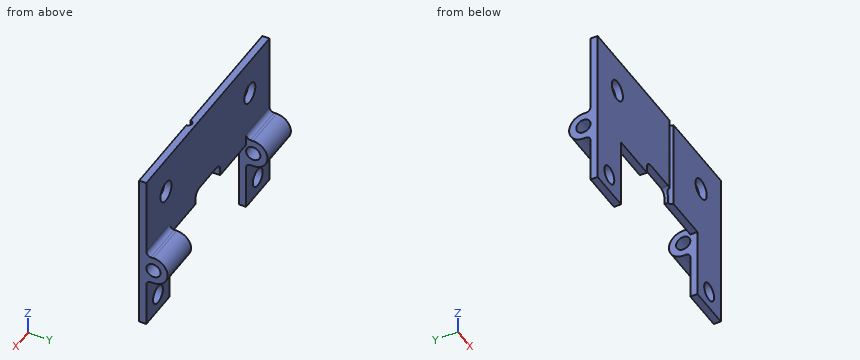
from build123d import *

# Parameters (mm, degrees)
SKETCH1_W                     = 25
SKETCH1_H                     = 10
BASE_PLATE_DEPTH              = 0.79
PINHOLDER_DEPTH               = 4.75
SKETCH4_R                     = 0.79
PIN_SHAFT_DEPTH               = 30.913269547
SKETCH5_R                     = 1.125
SCREW_HOLES_DEPTH             = 4
SKETCH11_R                    = 1
SET_SCREW_HOLE_DEPTH          = 1.5
MIRRORED_FILLETS_R            = 0.5
MIRRORED_FILLETS_OF_MIRROR1_R = 0.5
SKETCH9_RX                    = 0.4
SKETCH9_RY                    = 0.4
SKETCH10_W                    = 5
SKETCH10_H                    = 0.79
SPRING_GROOVE_DEPTH           = 1.5
FILLET2_R                     = 0.79


with BuildPart() as part:
    # Sketch1 → Base Plate (new body)
    with BuildSketch(Plane(origin=(0, 0, 0), x_dir=(1, 0, 0), z_dir=(0, 1, 0))):
        with Locations((1.323198198, 3.248873874)):
            Rectangle(SKETCH1_W, SKETCH1_H)
    extrude(amount=BASE_PLATE_DEPTH)

    # Sketch2 → PinHolder (add)
    with BuildSketch(Plane.ZY.offset(11.176801802)):
        with BuildLine():
            Line((-8.248873874, 0), (-8.248873874, 0.79))
            Line((-8.248873874, 0.79), (-7.458873874, 0.79))
            Line((-7.458873874, 0.79), (-7.458873874, 1.58))
            ThreePointArc((-7.458873874, 1.58), (-9.038873874, 3.16), (-10.618873874, 1.58))
            Line((-10.618873874, 1.58), (-10.618873874, 1.29))
            ThreePointArc((-10.618873874, 1.29), (-10.765320483, 0.936446609), (-11.118873874, 0.79))
            Line((-11.118873874, 0.79), (-16.118873874, 0.79))
            Line((-16.118873874, 0.79), (-16.118873874, 0))
            Line((-16.118873874, 0), (-11.426644498, 0))
            Line((-11.426644498, 0), (-8.248873874, 0))
        make_face()
    pinholder = extrude(amount=-PINHOLDER_DEPTH)

    # Sketch4 → Pin Shaft (cut, through all)
    with BuildSketch(Plane.ZY.offset(11.176801802)):
        with Locations((-9.038873874, 1.58)):
            Circle(SKETCH4_R)
    pin_shaft = extrude(amount=-PIN_SHAFT_DEPTH, mode=Mode.SUBTRACT)

    # Sketch5 → Screw Holes (cut)
    with BuildSketch(Plane(origin=(0, 0.79, 0), x_dir=(1, 0, 0), z_dir=(0, 1, 0))):
        with Locations(Location((-7.176801802, 2.248873874, 0), (0, 0, 270))):
            Circle(SKETCH5_R)
        with Locations(Location((9.823198198, 2.248873874, 0), (0, 0, 270))):
            Circle(SKETCH5_R)
    extrude(amount=-SCREW_HOLES_DEPTH, mode=Mode.SUBTRACT)

    # Sketch11 → Set Screw Hole (cut)
    with BuildSketch(Plane(origin=(0, 0.79, 0), x_dir=(1, 0, 0), z_dir=(0, 1, 0))):
        with Locations(Location((-8.801801802, 14.118873874, 0), (0, 0, 270))):
            Circle(SKETCH11_R)
    set_screw_hole = extrude(amount=-SET_SCREW_HOLE_DEPTH, mode=Mode.SUBTRACT)

    # Mirrored Fillets
    mirrored_fillets_edges = [part.edges().sort_by_distance(p)[0] for p in [
        (-8.801801802, 0.79, -7.458873874),
    ]]
    fillet(mirrored_fillets_edges, radius=MIRRORED_FILLETS_R)

    # Mirror1: PinHolder, Pin Shaft, Set Screw Hole across plane
    add(pinholder.mirror(Plane(origin=(1.323198198, 0, 0), x_dir=(0, 0, 1), z_dir=(1, 0, 0))))
    add(pin_shaft.mirror(Plane(origin=(1.323198198, 0, 0), x_dir=(0, 0, 1), z_dir=(1, 0, 0))), mode=Mode.SUBTRACT)
    add(set_screw_hole.mirror(Plane(origin=(1.323198198, 0, 0), x_dir=(0, 0, 1), z_dir=(1, 0, 0))), mode=Mode.SUBTRACT)

    # Mirrored Fillets of Mirror1
    mirrored_fillets_of_mirror1_edges = [part.edges().sort_by_distance(p)[0] for p in [
        (11.448198198, 0.79, -7.458873874),
    ]]
    fillet(mirrored_fillets_of_mirror1_edges, radius=MIRRORED_FILLETS_OF_MIRROR1_R)

    # Wire Groove: sweep along a path in Sketch8
    with BuildLine(Plane.XZ) as wire_groove_path:
        Line((3.823198198, -8.248873874), (3.823198198, 1.751126126))
    # Sketch9 → Wire Groove (sweep, cut)
    with BuildSketch(Plane.XY.offset(1.751126126)):
        with Locations((3.823198198, 0)):
            Ellipse(SKETCH9_RX, SKETCH9_RY)
    sweep(path=wire_groove_path.line, mode=Mode.SUBTRACT)

    # Sketch10 → Spring Groove (cut)
    with BuildSketch(Plane(origin=(0, 0, -8.248873874), x_dir=(-1, 0, 0), z_dir=(0, 0, -1))):
        with Locations((-1.323198198, 0.395)):
            Rectangle(SKETCH10_W, SKETCH10_H)
    extrude(amount=-SPRING_GROOVE_DEPTH, mode=Mode.SUBTRACT)

    # Fillet2
    fillet2_edges = [part.edges().sort_by_distance(p)[0] for p in [
        (-1.176801802, 0.395, -6.748873874),
        (3.823198198, 0.595, -6.748873874),
    ]]
    fillet(fillet2_edges, radius=FILLET2_R)


solid = part.part
Input: part model. Units: mm. Frame: model coordinates. Give positions to 0.01 mm unless a question says otherwise; leave off trailing zeros. Order: outer loops, then holes, each group sorted by start corner. A loop starts at its lowest first (then second) coordinate and runs counter-clockwise, first axis right, second up. Notation, with made-up numbers: (22, 41) - (64, 41) arc R19 ccw to (64, 58) - close; hole circle Ø1 at (39, -27.5). An arc over 180 degrees is marked (long way). Write each question's results on one line, items separated by ' | '.
Item 1: Section A-A (z = -14). Return loops of the section in (x, y).
A:
outline: (-11.18, 0) - (-9.79, 0) - (-9.79, 0.79) - (-11.18, 0.79) - close; (-7.81, 0) - (-6.43, 0) - (-6.43, 0.79) - (-7.81, 0.79) - close; (9.07, 0) - (10.46, 0) - (10.46, 0.79) - (9.07, 0.79) - close; (12.44, 0) - (13.82, 0) - (13.82, 0.79) - (12.44, 0.79) - close
Item 2: Section C-C (x = 0.5). Return loops of the section in (y, z), and give its area (4 significant figures).
A:
outline: (0, -6.75) - (0.79, -6.75) - (0.79, 1.75) - (0, 1.75) - close | area: 6.715 mm^2
Item 3: Section B-B (y = 1.85). Return loops of the section in (x, z), and give its area (3 significant figures).
A:
outline: (-11.18, -10.6) - (-6.43, -10.6) - (-6.43, -9.78) - (-11.18, -9.78) - close; (-11.18, -8.3) - (-6.43, -8.3) - (-6.43, -7.48) - (-11.18, -7.48) - close; (9.07, -10.6) - (13.82, -10.6) - (13.82, -9.78) - (9.07, -9.78) - close; (9.07, -8.3) - (13.82, -8.3) - (13.82, -7.48) - (9.07, -7.48) - close | area: 15.5 mm^2
Item 4: Contact query for flat-ended pins moving along their axis: pin 1 Ø3 at (x, z) = (2.5, -3) entering from +Y; pin 2 Ø1.5 at (x, y) = (11.5, 2.5) entering from -Z; pin 3 Ø0.9 at (x, y) = (-5, 0.5) entering from -Z. Output: stop coordinate, or through.
A:
pin 1: stops at y = 0.79 | pin 2: stops at z = -10.61 | pin 3: stops at z = -8.25
Item 5: Material intervals for line 1 along X through (y, z) = (2.75, -8.25); line 2 along Z through (x, y) = (-8.25, 1.6); line 3 along X through (y, z) = (0.35, -13.25), sorted ascending.
A:
line 1: x = -11.18 to -6.43, 9.07 to 13.82 | line 2: z = -10.62 to -9.83, -8.25 to -7.46 | line 3: x = -11.18 to -9.3, -8.31 to -6.43, 9.07 to 10.95, 11.94 to 13.82
Item 6: Section D-D (z = -3). Give the number of separate pieces and of enclosed holes in the cut face, and give its area (3 significant figures).
A:
separate pieces: 3 | enclosed holes: 0 | area: 16.9 mm^2
